Build history of the part. All positions in model axes, mm. Give positions to 0.01 mm unless a question says otherwise; leave off trailing zeros. Order: outer loops, then holes, each group sorted by start corner. A loop starts at its lowest first (then second) coordinate and runs counter-clockwise, first axis right, second up. Notation, with made-up numbers: (41, -14) - (69, -14) arc R11 cw to (69, 0) - close; hole circle Ø11 at (86, -29). An arc over 180 degrees is marked (long way). Answer in a Markdown table with one row per item.
```python
from build123d import *

# Parameters (mm, degrees)
BOSS_EXTRUDE1_DEPTH = 7.4
SKETCH2_R           = 3.983716857
BOSS_EXTRUDE2_DEPTH = 2.3
SKETCH3_R           = 2
BOSS_EXTRUDE3_DEPTH = 6
SKETCH4_R           = 0.5
BOSS_EXTRUDE4_DEPTH = 285


with BuildPart() as part:
    # Sketch1 → Boss-Extrude1 (new body)
    with BuildSketch(Plane.XY):
        Polygon((2.3, -3.983716857), (4.6, 0), (2.3, 3.983716857), (-2.3, 3.983716857), (-4.6, 0), (-2.3, -3.983716857), align=None)
    extrude(amount=BOSS_EXTRUDE1_DEPTH)

    # Sketch2 → Boss-Extrude2 (add)
    with BuildSketch(Plane.XY.offset(7.4)):
        Circle(SKETCH2_R)
    extrude(amount=BOSS_EXTRUDE2_DEPTH)

    # Sketch3 → Boss-Extrude3 (add)
    with BuildSketch(Plane.XY.offset(9.7)):
        Circle(SKETCH3_R)
    extrude(amount=BOSS_EXTRUDE3_DEPTH)

    # Sketch4 → Boss-Extrude4 (add)
    with BuildSketch(Plane.XY.offset(15.7)):
        Circle(SKETCH4_R)
    extrude(amount=BOSS_EXTRUDE4_DEPTH)


solid = part.part
```
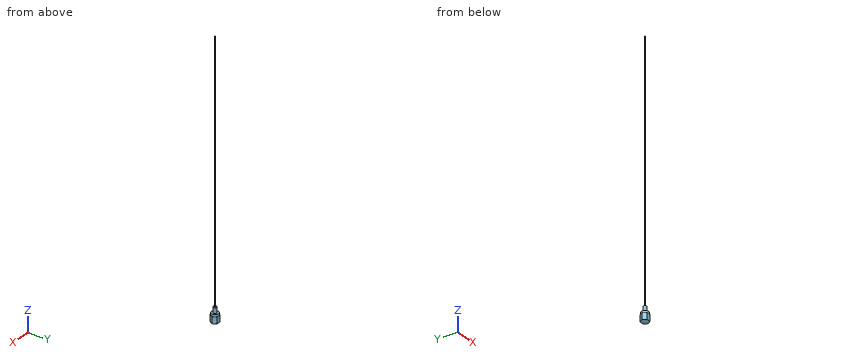
1. Cut at A-A on z = 138. Write the cut outline in (x, y).
Check result:
| item | result |
|---|---|
| outline | circle Ø1 at (0, 0) |
2. Probe line 1 (Z direction, x = 3.5, y = -0.5); line 2 (Z direction, x = -1.25, y = -1). List the from-to ranges inside material, lowest first.
Check result:
| item | result |
|---|---|
| line 1 | z = 0 to 9.7 |
| line 2 | z = 0 to 15.7 |
3. Drop flat-ended pins along their axis: P1, Ø2, axis at x = -1, y = -0.5, coming from the +Z side; P2, Ø1.3, axis at x = 4, y = -1, coming from the +Z side; P3, Ø2, axis at x = -0.5, y = -1.5, coming from the +Z side. Give the stop position or say it passes through.
Check result:
| item | result |
|---|---|
| P1 | stops at z = 300.7 |
| P2 | stops at z = 9.7 |
| P3 | stops at z = 15.7 |
